Input: part model. Units: mm. Frame: model coordinates. Face numbers are marked on the shaded views. A direction names the side the tool comes from. Round coordinates to 2 decimals unless told otherwise and drop trailing zeros. Write each loop counter-clockwise with the first axis right and the second up, starting at its lowest first coordinate (ties: lowest second). Pieces come first, ordered by that corner, then holes. Notation, with made-up numbers: (62, 59) -> (80, 59) arc R8 ccw to (80, 70) -> close; hole circle Ø7 at (-21, 2.25). An arc over 180 degrees is marked (long way). Use CSV: the item, a comma, the result in double quotes.
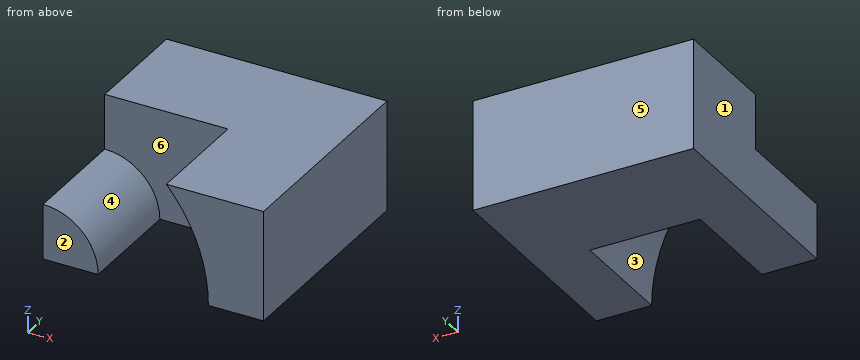
```python
from build123d import *

# Parameters (mm, degrees)
SKETCH_1_W    = 20
SKETCH_1_H    = 20
BASEBOX_DEPTH = 10
SKETCH_2_W    = 10
SKETCH_2_H    = 10


with BuildPart() as part:
    # 草图1 → BaseBox (new body)
    with BuildSketch(Plane.XY):
        with Locations((10, 10)):
            Rectangle(SKETCH_1_W, SKETCH_1_H)
    extrude(amount=BASEBOX_DEPTH)

    # 草图2 → RevolveCut360 (revolve, cut)
    with BuildSketch(Plane.XY):
        with Locations((10, 5)):
            Rectangle(SKETCH_2_W, SKETCH_2_H)
    revolve(axis=Axis((0, 0, 0), (0, 1, 0)), mode=Mode.SUBTRACT)


solid = part.part
```
Item 1: Line query: line 1 (Y direction, x = 12, z = 7); line 2 (X direction, y = 7.25, z = 3.25); line 3 (X direction, y = 1.75, z = 4). Output: solid intervals per line, ascending.
Worked answers:
line 1,"y = 10 to 20"
line 2,"x = 0 to 3.8, 14.64 to 20"
line 3,"x = 0 to 3, 14.46 to 20"
Item 2: Section query A-A on y = 9.5. Return the cut outline in (x, z), plus the area to 3 significant figures.
Worked answers:
outline,"(0, 0) -> (5, 0) arc R5 ccw to (0, 5) -> close; (11.18, 10) arc R15 cw to (15, 0) -> (20, 0) -> (20, 10) -> close"
area,"81.6 mm²"
Item 3: Section query B-B on z = 4.5. Return the cut outline in (x, y).
Worked answers:
outline,"(0, 0) -> (2.18, 0) -> (2.18, 10) -> (14.31, 10) -> (14.31, 0) -> (20, 0) -> (20, 20) -> (0, 20) -> close"
Item 4: Pull-direction query (X, two-part tool) for the marked faces 1, 2 and 3; classes: +X half, -X half, draft (parallel to the pull), parting line (faces both ways), or undercut.
Worked answers:
face 1,"-X half"
face 2,"draft"
face 3,"undercut"
Item 5: First-contact query: pin 1 Ø5 at (x, z) = (10.5, 6.5) entering from -Y. Flat tip, straight axial feed; report the tip coordinate or a pass-through.
Worked answers:
pin 1,"stops at y = 10"
Item 6: Section query C-C on x = 3. Return the cut outline in (y, z), plus the area to 3 significant figures.
Worked answers:
outline,"(0, 0) -> (20, 0) -> (20, 10) -> (10, 10) -> (10, 4) -> (0, 4) -> close"
area,"140 mm²"
Item 7: Section query D-D on z = 6.75. Return the cut outline in (x, y), plus the area to 3 significant figures.
Worked answers:
outline,"(0, 10) -> (13.4, 10) -> (13.4, 0) -> (20, 0) -> (20, 20) -> (0, 20) -> close"
area,"266 mm²"
Item 8: Set-up query: the marked faces 4, 5 and 6. Return all of +Z, -Z, +X, -X, +Y, -Y with unobstructed straight access to the full face (end or side cutting, diameter ignored); none if empty.
Worked answers:
face 4,"+Z, -Y"
face 5,"+Z, -Z, +X, -X, +Y"
face 6,"-Y"
